from build123d import *

# Parameters (mm, degrees)
F0_W      = 58.039
F0_H      = 14.605
F1_DEPTH  = 1.905
F2_W      = 1.905
F2_H      = 14.605
F3_DEPTH  = 26.035
F4_R      = 2.54
F6_DEPTH  = 58.04
F8_DEPTH  = 1.905
F10_DEPTH = 1.905
F12_DEPTH = 2.794
F14_DEPTH = 1.905
F16_DEPTH = 1.905


with BuildPart() as f1:
    # F0 (on Top) → F1 (new body)
    with BuildSketch(Plane.XY):
        Rectangle(F0_W, F0_H)
    extrude(amount=F1_DEPTH)

    # F2 (on face) → F3 (join)
    with BuildSketch(Plane.XY.offset(1.905)):
        with Locations((-28.067, 0)):
            Rectangle(F2_W, F2_H)
        with Locations((28.067, 0)):
            Rectangle(F2_W, F2_H)
    extrude(amount=F3_DEPTH)

    # F4
    f4_edges = [f1.edges().sort_by_distance(p)[0] for p in [
        (-29.0195, 0, 0),
        (29.0195, 0, 0),
        (27.1145, 0, 1.905),
        (-27.1145, 0, 1.905),
    ]]
    fillet(f4_edges, radius=F4_R)

    # F5 (on face) → F6 (cut, through all)
    with BuildSketch(Plane(origin=(-29.0195, 0, 0), x_dir=(0, -1, 0), z_dir=(-1, 0, 0))):
        with BuildLine():
            Line((3.175, 27.94), (-3.175, 27.94))
            ThreePointArc((-3.175, 27.94), (0, 24.765), (3.175, 27.94))
        make_face()
    extrude(amount=-F6_DEPTH, mode=Mode.SUBTRACT)

    # F7 (on face) → F8 (cut, through all)
    with BuildSketch(Plane.XY.offset(1.905)):
        with BuildLine():
            Line((-18.2245, 2.4257), (-19.4183, 2.4257))
            ThreePointArc((-19.4183, 2.4257), (-21.844, 0), (-19.4183, -2.4257))
            Line((-19.4183, -2.4257), (-18.2245, -2.4257))
            ThreePointArc((-18.2245, -2.4257), (-15.7988, 0), (-18.2245, 2.4257))
        make_face()
        with BuildLine():
            Line((19.4183, 2.4257), (18.2245, 2.4257))
            ThreePointArc((18.2245, 2.4257), (15.7988, 0), (18.2245, -2.4257))
            Line((18.2245, -2.4257), (19.4183, -2.4257))
            ThreePointArc((19.4183, -2.4257), (21.844, 0), (19.4183, 2.4257))
        make_face()
    extrude(amount=-F8_DEPTH, mode=Mode.SUBTRACT)

    # F9 (on face) → F10 (cut, through all)
    with BuildSketch(Plane.XY.offset(1.905)):
        Polygon((-7.3025, -2.413), (-19.4945, -7.3025), (19.4945, -7.3025), (7.3025, -2.413), align=None)
    extrude(amount=-F10_DEPTH, mode=Mode.SUBTRACT)

    # F11 (on face) → F12 (join)
    with BuildSketch(Plane.XY.offset(1.905)):
        Polygon((-20.2035866979, -5.5343877143), (-19.4945, -7.3025), (-7.3025, -2.413), (7.3025, -2.413), (19.4945, -7.3025), (20.2035866979, -5.5343877143), (7.6702562934, -0.508), (-7.6702562934, -0.508), align=None)
    extrude(amount=F12_DEPTH)

    # F13 (on face) → F14 (cut, through all)
    with BuildSketch(Plane(origin=(-0.1781303134, 0.4441690931, 0), x_dir=(0.9281429321, 0.3722239884, 0), z_dir=(0.3722239884, -0.9281429321, 0))):
        Polygon((-20.8118480657, 4.699), (-20.8118480657, 1.905), (-7.6759402459, 4.699), align=None)
    extrude(amount=-F14_DEPTH, mode=Mode.SUBTRACT)

    # F15 (on face) → F16 (cut, through all)
    with BuildSketch(Plane(origin=(0.1781303134, 0.4441690931, 0), x_dir=(0.9281429321, -0.3722239884, 0), z_dir=(-0.3722239884, -0.9281429321, 0))):
        Polygon((7.6759402459, 4.699), (20.8118480657, 1.905), (20.8118480657, 4.699), align=None)
    extrude(amount=-F16_DEPTH, mode=Mode.SUBTRACT)


solid = f1.part
Check sheet for the modelled part. Datum: model origin and axes. Units: mm. A direction names the side the tool comes from. Give positions to 0.01 mm unless a question says otherwise; leave off trailing zeros. Loops run counter-clockwise (first coordinate to the right, second up) from the corner with the lowest first, then second, coordinate; pieces in that order, holes last. Notation, with made-up numbers: M 89.5,60 L 124.5,60 A17 cw 124.5,93 Z; hole C 10.5,23 d1. An arc over 180 degrees is marked long. Answer as a JSON object with one key per item and string values. Group by question number.
Q1. Material ranges on line 1 along X through (y, z) = (2.5, 24.25); line 2 along Z through (x, y) = (1.5, -1.25); line 3 along Z through (x, y) = (3.5, 4) (3 decimals), recorded low to high. Write a range as [from, to].
Q2. Cross-section at A-A on z = 10.5. Record the cut outline in (x, y), then the cut area to 3 significant figures.
Q3. Access from +Z, -Z, +X, -X, +Y, -Y to the whole of each face (thin tool, end or side, straight path). Record for faces 4 (the cylindrical face through (-21.843, 0.053, 0.966)), 5 (the flat face through (-12.46, -2.43, 2.97)), 6 (the flat face through (0, -2.413, 2)).
Q4. Cross-section at B-B on y = 0.5. Record the cut outline in (x, z) (1 decimal).
Q5. Release check for a two-part mould opening along Y. For faces 1 (the cylindrical face through (28.295, 0.102, 0.764)), 2 (the cylindrical face through (-15.8, -0.1, 1)), 3 (the flat face through (11.96, -4.28, 1.79)) record: released by +Y, released by -Y, zero draft, split by the parting line, or undercut.
Q6. Cross-section at C-C on z = 3.75. Record the cut outline in (x, y).
Q7. Cross-section at D-D on y = 6.25. Record the cut outline in (x, z) (1 decimal), then the cut area to 3 significant figures.
Q8. Go/stop test with flat-tipped pins: P1, Ø0.8, axis at x = -1.5, z = 3.5, coming from the +Y side; P2, Ø4.5, axis at x = -2.5, y = 3, coming from the +Z side (3 decimals); P3, Ø1, axis at x = -18.5, z = 0.5, coming from the -Y side; P4, Ø6, axis at x = -12.5, y = -1, coming from the -Z side. Record where each tip stops, or that it passes through.
Evaluation:
{
 "1": {"line 1": "x = [-29.02, -27.11], [27.11, 29.02]", "line 2": "z = [0, 4.7]", "line 3": "z = [0, 1.905]"},
 "2": {"outline": "M -29.02,-7.3 L -27.11,-7.3 L -27.11,7.3 L -29.02,7.3 Z; M 27.11,-7.3 L 29.02,-7.3 L 29.02,7.3 L 27.11,7.3 Z", "area": "55.6 mm2"},
 "3": {"face 4": "+Z, -Z", "face 5": "+Z, +Y", "face 6": "+Z, -Z, -Y"},
 "4": {"outline": "M -29,2.5 A2.5 ccw -26.5,0 L -21.8,0 L -21.8,1.9 L -24.6,1.9 A2.5 cw -27.1,4.4 L -27.1,24.8 L -29,24.8 Z; M -15.9,0 L 15.9,0 L 15.9,1.9 L -15.9,1.9 Z; M 21.8,0 L 26.5,0 A2.5 ccw 29,2.5 L 29,24.8 L 27.1,24.8 L 27.1,4.4 A2.5 cw 24.6,1.9 L 21.8,1.9 Z"},
 "5": {"face 1": "zero draft", "face 2": "undercut", "face 3": "released by -Y"},
 "6": {"outline": "M -29.02,-7.3 L -27.02,-7.3 L -27.02,7.3 L -29.02,7.3 Z; M -12.15,-2.31 L -11.44,-4.07 L -7.3,-2.41 L 7.3,-2.41 L 11.44,-4.07 L 12.15,-2.31 L 7.67,-0.51 L -7.67,-0.51 Z; M 27.02,-7.3 L 29.02,-7.3 L 29.02,7.3 L 27.02,7.3 Z"},
 "7": {"outline": "M -29,2.5 A2.5 ccw -26.5,0 L 26.5,0 A2.5 ccw 29,2.5 L 29,27.9 L 27.1,27.9 L 27.1,4.4 A2.5 cw 24.6,1.9 L -24.6,1.9 A2.5 cw -27.1,4.4 L -27.1,27.9 L -29,27.9 Z", "area": "210 mm2"},
 "8": {"P1": "stops at y = -0.51", "P2": "stops at z = 1.905", "P3": "stops at y = -7.1", "P4": "stops at z = 0"}
}
